Could you check a few things on this model? Use its own coordinates, in mm. Face numbers are marked on the shaded views. A direction names the side the tool comes from. Round coordinates to 2 decimals unless told otherwise and drop trailing zeros. Loops run counter-clockwise (first coordinate to the right, second up) from the corner with the lowest first, then second, coordinate; pieces in that order, holes last. Notation, with made-up numbers: (41, -32.75) -> (66, -32.75) arc R15 cw to (66, -17.75) -> close; hole circle Ø3 at (-24.5, -31.5). An arc over 180 degrees is marked (long way). One line per item, written item: value.
```python
from build123d import *

# Parameters (mm, degrees)
SKETCH1_R           = 1.3335
SKETCH1_R_2         = 1.5875
BOSS_EXTRUDE1_DEPTH = 1.651
CHAMFER1_SIZE       = 2.54
SKETCH1_2_R         = 1.5875
BOSS_EXTRUDE2_DEPTH = 2.413
SKETCH1_3_R         = 1.5875
CUT_EXTRUDE1_DEPTH  = 0.889
CUT_EXTRUDE2_DEPTH  = 23.382376376


with BuildPart() as part:
    # Sketch1 → Boss-Extrude1 (new body)
    with BuildSketch(Plane(origin=(0, 0, 0), x_dir=(1, 0, 0), z_dir=(0, 1, 0))):
        with BuildLine():
            Line((-5.567119422, 8.9535), (5.567119422, 8.9535))
            ThreePointArc((5.567119422, 8.9535), (6.35, 6.5405), (7.132880578, 8.9535))
            Line((7.132880578, 8.9535), (20.447, 8.9535))
            Line((20.447, 8.9535), (20.447, -8.9535))
            Line((20.447, -8.9535), (7.132880578, -8.9535))
            ThreePointArc((7.132880578, -8.9535), (6.35, -6.5405), (5.567119422, -8.9535))
            Line((5.567119422, -8.9535), (-5.567119422, -8.9535))
            ThreePointArc((-5.567119422, -8.9535), (-6.35, -6.5405), (-7.132880578, -8.9535))
            Line((-7.132880578, -8.9535), (-20.447, -8.9535))
            Line((-20.447, -8.9535), (-20.447, 8.9535))
            Line((-20.447, 8.9535), (-7.132880578, 8.9535))
            ThreePointArc((-7.132880578, 8.9535), (-6.35, 6.5405), (-5.567119422, 8.9535))
        make_face()
        with Locations(Location((-17.8308, 5.6769, 0), (0, 0, 90))):
            Circle(SKETCH1_R, mode=Mode.SUBTRACT)
        with Locations(Location((17.8308, 5.6769, 0), (0, 0, 90))):
            Circle(SKETCH1_R, mode=Mode.SUBTRACT)
        with Locations(Location((17.8308, -5.6769, 0), (0, 0, 90))):
            Circle(SKETCH1_R, mode=Mode.SUBTRACT)
        with Locations(Location((-17.8308, -5.6769, 0), (0, 0, 90))):
            Circle(SKETCH1_R, mode=Mode.SUBTRACT)
        with Locations(Location((-10.414, 5.6769, 0), (0, 0, 90))):
            Circle(SKETCH1_R_2, mode=Mode.SUBTRACT)
        with Locations(Location((10.414, 5.6769, 0), (0, 0, 90))):
            Circle(SKETCH1_R_2, mode=Mode.SUBTRACT)
        with Locations(Location((10.414, -5.6769, 0), (0, 0, 90))):
            Circle(SKETCH1_R_2, mode=Mode.SUBTRACT)
        with Locations(Location((-10.414, -5.6769, 0), (0, 0, 90))):
            Circle(SKETCH1_R_2, mode=Mode.SUBTRACT)
    extrude(amount=BOSS_EXTRUDE1_DEPTH)

    # Chamfer1
    chamfer1_edges = [part.edges().sort_by_distance(p)[0] for p in [
        (20.447, 0.8255, -8.9535),
        (20.447, 0.8255, 8.9535),
        (-20.447, 0.8255, 8.9535),
        (-20.447, 0.8255, -8.9535),
    ]]
    chamfer(chamfer1_edges, length=CHAMFER1_SIZE)

    # Sketch1_2 → Boss-Extrude2 (add)
    with BuildSketch(Plane(origin=(0, 0, 0), x_dir=(1, 0, 0), z_dir=(0, 1, 0))):
        with Locations(Location((-10.414, 5.6769, 0), (0, 0, 270))):
            Circle(SKETCH1_2_R)
        with Locations(Location((10.414, 5.6769, 0), (0, 0, 270))):
            Circle(SKETCH1_2_R)
        with Locations(Location((10.414, -5.6769, 0), (0, 0, 270))):
            Circle(SKETCH1_2_R)
        with Locations(Location((-10.414, -5.6769, 0), (0, 0, 270))):
            Circle(SKETCH1_2_R)
    extrude(amount=BOSS_EXTRUDE2_DEPTH)

    # Sketch1_3 → Cut-Extrude1 (cut)
    with BuildSketch(Plane(origin=(0, 0, 0), x_dir=(1, 0, 0), z_dir=(0, 1, 0))):
        with Locations(Location((-10.414, 5.6769, 0), (0, 0, 270))):
            Circle(SKETCH1_3_R)
        with Locations(Location((10.414, 5.6769, 0), (0, 0, 270))):
            Circle(SKETCH1_3_R)
        with Locations(Location((10.414, -5.6769, 0), (0, 0, 270))):
            Circle(SKETCH1_3_R)
        with Locations(Location((-10.414, -5.6769, 0), (0, 0, 270))):
            Circle(SKETCH1_3_R)
    extrude(amount=CUT_EXTRUDE1_DEPTH, mode=Mode.SUBTRACT)

    # Sketch2 → Cut-Extrude2 (cut, through all)
    with BuildSketch(Plane(origin=(0, 1.651, 0), x_dir=(1, 0, 0), z_dir=(0, 1, 0))):
        with BuildLine():
            Line((-10.033, 1.5875), (-10.033, 1.630758795))
            Line((-10.033, 1.630758795), (-12.339241205, 3.937))
            Line((-12.339241205, 3.937), (-15.600758795, 3.937))
            Line((-15.600758795, 3.937), (-17.907, 1.630758795))
            Line((-17.907, 1.630758795), (-17.907, -1.630758795))
            Line((-17.907, -1.630758795), (-15.600758795, -3.937))
            Line((-15.600758795, -3.937), (-12.339241205, -3.937))
            Line((-12.339241205, -3.937), (-10.033, -1.630758795))
            Line((-10.033, -1.630758795), (-10.033, -1.5875))
            Line((-10.033, -1.5875), (-6.279440481, -1.5875))
            ThreePointArc((-6.279440481, -1.5875), (0, -6.477), (6.279440481, -1.5875))
            Line((6.279440481, -1.5875), (10.033, -1.5875))
            Line((10.033, -1.5875), (10.033, -1.630758795))
            Line((10.033, -1.630758795), (12.339241205, -3.937))
            Line((12.339241205, -3.937), (15.600758795, -3.937))
            Line((15.600758795, -3.937), (17.907, -1.630758795))
            Line((17.907, -1.630758795), (17.907, 1.630758795))
            Line((17.907, 1.630758795), (15.600758795, 3.937))
            Line((15.600758795, 3.937), (12.339241205, 3.937))
            Line((12.339241205, 3.937), (10.033, 1.630758795))
            Line((10.033, 1.630758795), (10.033, 1.5875))
            Line((10.033, 1.5875), (6.279440481, 1.5875))
            ThreePointArc((6.279440481, 1.5875), (0, 6.477), (-6.279440481, 1.5875))
            Line((-6.279440481, 1.5875), (-10.033, 1.5875))
        make_face()
    extrude(amount=-CUT_EXTRUDE2_DEPTH, mode=Mode.SUBTRACT)


solid = part.part
```
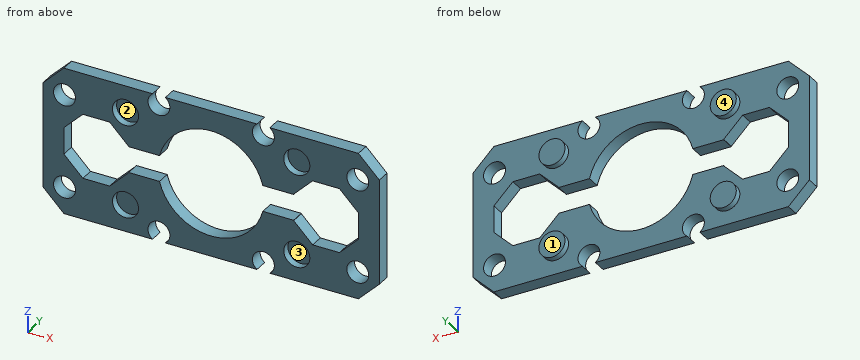
(1) Imagine slicing it at D-D on z = 5.75. Give the number of separate pieces and of enclosed holes in the cut face, then the cut area to 3 significant figures.
Results below:
separate pieces: 4
enclosed holes: 0
area: 48.1 mm²
(2) Imagine slicing it at B-B on x = -2. Write out the boundary of the cut face in (y, z).
Results below:
outline: (0, -8.95) -> (1.65, -8.95) -> (1.65, -6.16) -> (0, -6.16) -> close; (0, 6.16) -> (1.65, 6.16) -> (1.65, 8.95) -> (0, 8.95) -> close
(3) For pin 1 Ø4.5 at (x, z) = (-6.35, -7.874) entering from +Y; pin 2 Ø3.5 at (x, z) = (-10.41, -5.68) entering from -Y; pin 3 Ø1 at (x, z) = (11, 5) entering from -Y, each with a flat end and sliding along its axis, tell me the tip position at first contact or that it passes through.
Results below:
pin 1: stops at y = 1.65
pin 2: stops at y = 0
pin 3: stops at y = 0.89
(4) We'd pull the mould along X, two halves only. Please class the marked faces 1 and 2: +X half, -X half, draft (parallel to the pull), parting line (faces both ways), or undercut.
Results below:
face 1: draft
face 2: undercut
(5) Imagine slicing it at C-C on z = -2.5. Write out the boundary of the cut face in (x, y), then the cut area to 3 significant figures.
Results below:
outline: (-20.45, 0) -> (-17.04, 0) -> (-17.04, 1.65) -> (-20.45, 1.65) -> close; (-10.9, 0) -> (-5.98, 0) -> (-5.98, 1.65) -> (-10.9, 1.65) -> close; (5.98, 0) -> (10.9, 0) -> (10.9, 1.65) -> (5.98, 1.65) -> close; (17.04, 0) -> (20.45, 0) -> (20.45, 1.65) -> (17.04, 1.65) -> close
area: 27.5 mm²
(6) Please list where these lines run through material, in increasing order: L1, parallel to X at y = 0.8, z = 0.5; L2, parallel to Z at x = 18, y = 1.2; L3, parallel to X at y = 0.8, z = 7.5.
Results below:
L1: x = -20.45 to -17.91, 17.91 to 20.45
L2: z = -8.86 to -7, -4.35 to 4.35, 7 to 8.86
L3: x = -19.36 to -7.63, -5.07 to 5.07, 7.63 to 19.36
(7) Imagine slicing it at A-A on z = 0.25. Write out the boundary of the cut face in (x, y).
Results below:
outline: (-20.45, 0) -> (-17.91, 0) -> (-17.91, 1.65) -> (-20.45, 1.65) -> close; (17.91, 0) -> (20.45, 0) -> (20.45, 1.65) -> (17.91, 1.65) -> close
(8) On a 3-axis mill with a long thin cutter (end or side, diameter ignored), from which of +Z, -Z, +X, -X, +Y, -Y can I reach the whole of each face in a straight line? I mean the marked faces 3 and 4. Say none if no direction works.
Results below:
face 3: -Y
face 4: +Z, -Z, +X, -X, +Y
